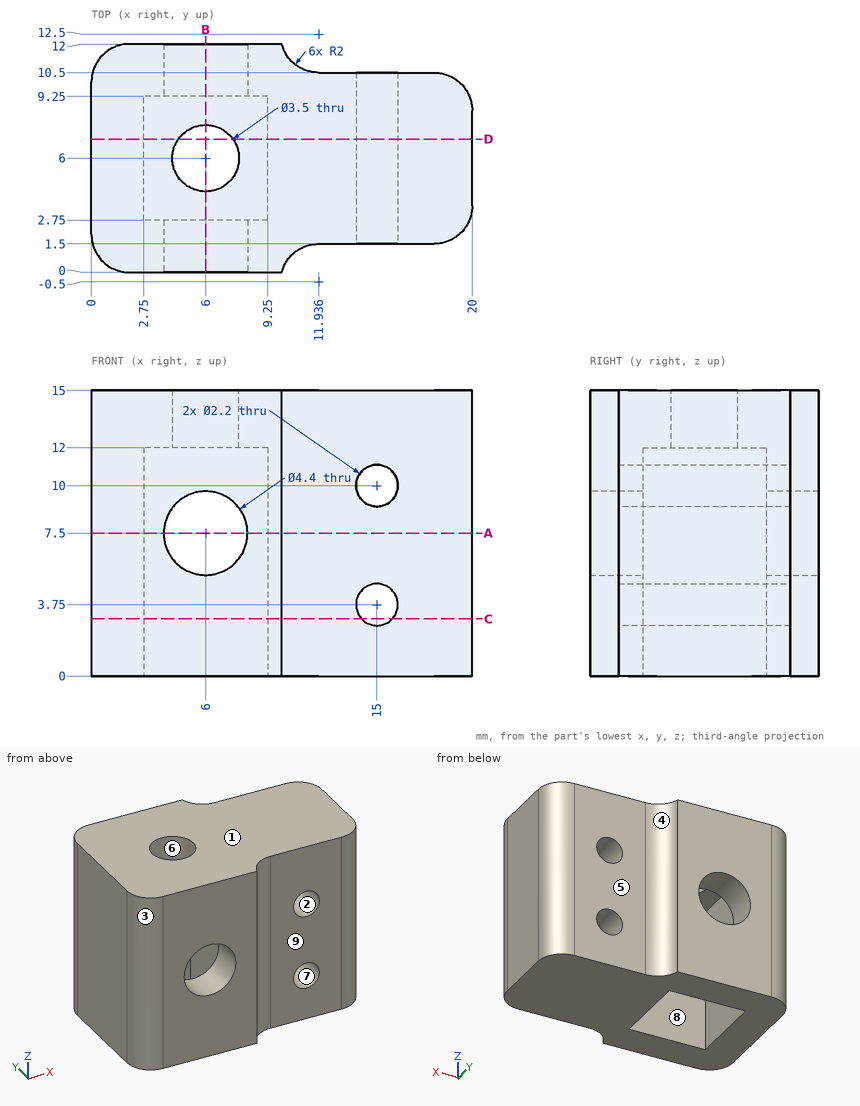
Here's the drawing with two shaded views (mm, measured from the low corner). I have some questions. A direction names the side the tool comes from. Coordinates: 2 decimals unless noted, no trailing zeros. Order: outer loops, then holes, each group sorted by start corner. A loop starts at its lowest first (then second) coordinate and runs counter-clockwise, first axis right, second up.
Q1. Please list where these lines run through material, in increasing order: L1, parallel to X at y = 5, z = 3.75; L2, parallel to Y at x = 3, z = 7; L3, parallel to Y at x = 6, z = 13.7.
Q2. Suppose I cut it at A-A on z = 7.5. Please give me the cut outline in (x, y), and give its area (3 significant figures).
Q3. Which directions (+Z, -Z, +X, -X, +Y, -Y) give clear straight access to the entire face, cutting with the end or side of a thin tool? Please do the marked faces 5, 6, 7, 8 and 9.
Q4. Suppose I cut it at B-B on x = 6. Please give me the cut outline in (y, z).
Q5. Will these pins go through, and if not, where does the flat tip stop? pin 1 (2.5 mm diameter, centred on x = 6, z = 7.5, fed in from -Y); pin 2 (5 mm diameter, centred on x = 16.5, z = 4.5, fed in from +Y); pin 3 (3.5 mm diameter, centred on x = 15, z = 3.75, fed in from -Y); pin 4 (3 mm diameter, centred on x = 7, y = 7.5, fed in from -Z).
Q6. Thinking about a two-plate mould opening in X: for the marked faces 1, 2, 3 and 4, which applies, released by +X, released by -X, zero draft, split by the parting line, or undercut?
Q7. Suppose I cut it at C-C on z = 3. Give the number of separate pieces and of enclosed holes in the cut face, and give its area (3 significant figures).
Q8. Suppose I cut it at D-D on y = 7. Please give me the cut outline in (x, z), and give its area (3 significant figures).
Answer:
1. L1: x = 0 to 2.75, 9.25 to 13.9, 16.1 to 20
1. L2: y = 0 to 2.75, 9.25 to 12
1. L3: y = 0 to 4.25, 7.75 to 12
2. outline: (0, 2) arc R2 ccw to (2, 0) - (3.8, 0) - (3.8, 2.75) - (2.75, 2.75) - (2.75, 9.25) - (3.8, 9.25) - (3.8, 12) - (2, 12) arc R2 ccw to (0, 10) - close; (8.2, 0) - (10, 0) arc R2 cw to (11.94, 1.5) - (18, 1.5) arc R2 ccw to (20, 3.5) - (20, 8.5) arc R2 ccw to (18, 10.5) - (11.94, 10.5) arc R2 cw to (10, 12) - (8.2, 12) - (8.2, 9.25) - (9.25, 9.25) - (9.25, 2.75) - (8.2, 2.75) - close
2. area: 142 mm2
3. face 5: +Z, -Z, +X, +Y
3. face 6: +Z, -Z
3. face 7: +Y, -Y
3. face 8: -Z
3. face 9: +Z, -Z, +X, -Y
4. outline: (0, 0) - (2.75, 0) - (2.75, 5.3) - (0, 5.3) - close; (0, 9.7) - (2.75, 9.7) - (2.75, 12) - (4.25, 12) - (4.25, 15) - (0, 15) - close; (7.75, 12) - (9.25, 12) - (9.25, 9.7) - (12, 9.7) - (12, 15) - (7.75, 15) - close; (9.25, 0) - (12, 0) - (12, 5.3) - (9.25, 5.3) - close
5. pin 1: passes through
5. pin 2: stops at y = 10.5
5. pin 3: stops at y = 1.5
5. pin 4: stops at z = 12
6. face 1: zero draft
6. face 2: undercut
6. face 3: released by -X
6. face 4: released by +X
7. separate pieces: 2
7. enclosed holes: 1
7. area: 151 mm2
8. outline: (0, 0) - (2.75, 0) - (2.75, 12) - (4.56, 12) - (4.56, 15) - (0, 15) - close; (7.44, 12) - (9.25, 12) - (9.25, 0) - (20, 0) - (20, 15) - (7.44, 15) - close; hole circle Ø2.2 at (15, 3.75); hole circle Ø2.2 at (15, 10)
8. area: 206 mm2
